Check sheet for the modelled part. Datum: model origin and axes. Units: mm. Face numbers are marked on the shaded views. A direction names the side the tool comes from. Give positions to 0.01 mm unless a question says otherwise; leave off trailing zeros. Write each loop counter-clockwise with the first axis right and the second up, starting at its lowest first coordinate (ties: lowest second). Pieces come first, ordered by that corner, then holes. Notation, with made-up numbers: M 68,23 L 89,23 A17 cw 89,54 Z; hole C 31,-19 d4. An arc over 180 degrees is marked long. Write item = value, one per line. Start each with the question number.
1) Scan lines: line 1 along Z through (x, y) = (20.5, 6.25); line 2 along Z through (x, y) = (18, 1.75); line 3 along Z through (x, y) = (66, 1.5). Record each from-to range of solid material in increasing order. Write a range as [from, to].
2) Cross-section at A-A, the plane x = 63.5. Record the cut outline in (y, z), plus the area to 3 significant figures.
3) Cross-section at B-B, the plane y = 2.5. Record the cut outline in (x, z).
4) Mould release check, pull along Z, two halves, no side actions. Record for the marked faces 1, 2 and 3: released by +Z, released by -Z, zero draft, split by the parting line, or undercut.
5) Cross-section at C-C, the plane z = -9. Record the cut outline in (x, y).
6) Go/stop test with flat-tipped pins: pin 1 (1.9 mm diameter, centred on y = 8.5, z = 12, fed in from +X); pin 2 (1.1 mm diameter, centred on x = -80, z = 13.5, fed in from +Y). Record where each tip stops, or that it passes through.
7) Access from +Z, -Z, +X, -X, +Y, -Y to the whole of each face (thin tool, end or side, straight path). Record for the marked faces 4 and 5.
8) Cross-section at D-D, the plane x = 41.5. Record the cut outline in (y, z).
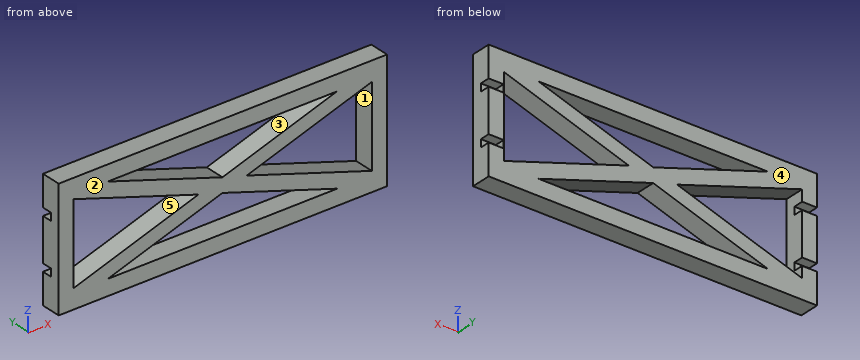
```python
from build123d import *

# Parameters (mm, degrees)
SKETCH1_W           = 165
SKETCH1_H           = 60
BOSS_EXTRUDE1_DEPTH = 10
SKETCH2_W           = 3.81
SKETCH2_H           = 5
CUT_EXTRUDE1_DEPTH  = 7.5


with BuildPart() as part:
    # Sketch1 → Boss-Extrude1 (new body)
    with BuildSketch(Plane(origin=(0, 0, 0), x_dir=(1, 0, 0), z_dir=(0, 1, 0))):
        Rectangle(SKETCH1_W, SKETCH1_H)
        Polygon((-75.04, 20.262432489), (-75.04, -20.262432489), (-12.226459283, 0), align=None, mode=Mode.SUBTRACT)
        Polygon((57.460458264, 22.165834991), (-57.834623171, 22.165834991), (-0.187082453, 3.569854115), align=None, mode=Mode.SUBTRACT)
        Polygon((74.852917547, 20.262432489), (74.852917547, -20.262432489), (12.039376829, 0), align=None, mode=Mode.SUBTRACT)
        Polygon((-57.834623171, -22.165834991), (-0.187082453, -3.569854115), (57.460458264, -22.165834991), align=None, mode=Mode.SUBTRACT)
    extrude(amount=BOSS_EXTRUDE1_DEPTH)

    # Sketch2 → Cut-Extrude1 (cut)
    with BuildSketch(Plane.ZY.offset(82.5)):
        with Locations((-12.7, 7.5)):
            Rectangle(SKETCH2_W, SKETCH2_H)
        with Locations((12.7, 7.5)):
            Rectangle(SKETCH2_W, SKETCH2_H)
    cut_extrude1 = extrude(amount=-CUT_EXTRUDE1_DEPTH, mode=Mode.SUBTRACT)

    # Mirror1: Cut-Extrude1 across plane
    add(cut_extrude1.mirror(Plane(origin=(0, 0, 0), x_dir=(0, 0, 1), z_dir=(1, 0, 0))), mode=Mode.SUBTRACT)


solid = part.part
```
Reply:
q1.line_1 = [-30, -22.17], [-10.24, -2.73], [2.73, 10.24], [22.17, 30]
q1.line_2 = [-30, -22.17], [-9.44, -1.92], [1.92, 9.44], [22.17, 30]
q1.line_3 = [-30, -17.41], [17.41, 30]
q2.outline = M 0,-30 L 10,-30 L 10,-16.6 L 0,-16.6 Z; M 0,16.6 L 10,16.6 L 10,30 L 0,30 Z
q2.area = 268 mm2
q3.outline = M -82.5,-30 L 82.5,-30 L 82.5,30 L -82.5,30 Z; hole M -75.04,-20.26 L -12.23,0 L -75.04,20.26 Z; hole M -57.83,-22.17 L 57.46,-22.17 L -0.19,-3.57 Z; hole M -57.83,22.17 L -0.19,3.57 L 57.46,22.17 Z; hole M 12.04,0 L 74.85,-20.26 L 74.85,20.26 Z
q4.face_1 = undercut
q4.face_2 = zero draft
q4.face_3 = undercut
q5.outline = M -82.5,0 L -75.04,0 L -75.04,10 L -82.5,10 Z; M -40.13,0 L -17.02,0 L -17.02,10 L -40.13,10 Z; M 16.65,0 L 39.94,0 L 39.94,10 L 16.65,10 Z; M 74.85,0 L 82.5,0 L 82.5,10 L 74.85,10 Z
q6.pin_1 = 75
q6.pin_2 = 5
q7.face_4 = +Z, -Z, +X, -X, +Y
q7.face_5 = +Y, -Y
q8.outline = M 0,-30 L 10,-30 L 10,-22.17 L 0,-22.17 Z; M 0,-17.02 L 10,-17.02 L 10,-9.5 L 0,-9.5 Z; M 0,9.5 L 10,9.5 L 10,17.02 L 0,17.02 Z; M 0,22.17 L 10,22.17 L 10,30 L 0,30 Z
